```python
from build123d import *

# Parameters (mm, degrees)
SKETCH2_OUTSIDE_W = 12.738
SKETCH2_OUTSIDE_H = 12.738
EXTRUDE1_DEPTH    = 6
SKETCH3_R         = 2.125
EXTRUDE2_DEPTH    = 2
EXTRUDE2_TAPER    = 20
SKETCH4_R         = 1.35
EXTRUDE3_DEPTH    = 12
SKETCH5_W         = 1.5
SKETCH5_H         = 7.5
EXTRUDE4_DEPTH    = 0.75


with BuildPart() as part:
    # Sketch1 → Revolve1 (revolve)
    with BuildSketch(Plane.XY, mode=Mode.PRIVATE) as revolve1_sk:
        with BuildLine():
            Line((-6.597555333, -81.619969832), (-4.417555333, -81.619969832))
            ThreePointArc((-4.417555333, -81.619969832), (-4.276133977, -81.561391188), (-4.217555333, -81.419969832))
            Line((-4.217555333, -81.419969832), (-4.217555333, -80.780202359))
            ThreePointArc((-4.217555333, -80.780202359), (-4.241407579, -80.627613643), (-4.310688598, -80.489583262))
            Line((-4.310688598, -80.489583262), (-5.467555333, -78.869969832))
            Line((-5.467555333, -78.869969832), (-5.467555333, -72.569969832))
            Line((-5.467555333, -72.569969832), (-5.467555333, -68.619969832))
            Line((-5.467555333, -68.619969832), (-6.597555333, -68.619969832))
            Line((-6.597555333, -68.619969832), (-6.597555333, -81.619969832))
        make_face()
    revolve(revolve1_sk.sketch.rotate(Axis((-7.917555333, -68.619969832, 0), (0, -1, 0)), 180), axis=Axis((-7.917555333, -68.619969832, 0), (0, -1, 0)))

    # Sketch2 outside → Extrude1 (cut)
    with BuildSketch(Plane(origin=(0, -68.619969832, 0), x_dir=(-1, 0, 0), z_dir=(0, 1, 0))):
        with Locations((7.918, 0)):
            Rectangle(SKETCH2_OUTSIDE_W, SKETCH2_OUTSIDE_H)
        Polygon((5.301260243, 0), (7.917555333, -2.61629509), (10.533850424, 0), (7.917555333, 2.61629509), align=None, mode=Mode.SUBTRACT)
    extrude(amount=-EXTRUDE1_DEPTH, mode=Mode.SUBTRACT)

    # Sketch3 → Extrude2 (add)
    with BuildSketch(Plane(origin=(0, -74.619969832, 0), x_dir=(-1, 0, 0), z_dir=(0, 1, 0))):
        with Locations((7.917555333, 0)):
            Circle(SKETCH3_R)
    extrude(amount=EXTRUDE2_DEPTH, taper=EXTRUDE2_TAPER)

    # Sketch4 → Extrude3 (cut)
    with BuildSketch(Plane(origin=(0, -68.619969832, 0), x_dir=(-1, 0, 0), z_dir=(0, 1, 0))):
        with Locations((7.917555333, 0)):
            Circle(SKETCH4_R)
    extrude(amount=-EXTRUDE3_DEPTH, mode=Mode.SUBTRACT)

    # Sketch5 → Extrude4 (cut)
    with BuildSketch(Plane.XZ.offset(81.619969832)):
        with Locations((-7.917555333, 0)):
            Rectangle(SKETCH5_W, SKETCH5_H)
    extrude(amount=-EXTRUDE4_DEPTH, mode=Mode.SUBTRACT)


solid = part.part
```
Part model, mm, in its own coordinate system. A direction names the side the tool comes from. Round coordinates to 2 decimals unless told otherwise and drop trailing zeros. Write each loop counter-clockwise with the first axis right and the second up, starting at its lowest first coordinate (ties: lowest second). Pieces come first, ordered by that corner, then holes. Notation, with made-up numbers: (47.5, 86.25) -> (60.5, 86.25) arc R11 ccw to (60.5, 94.25) -> close; hole circle Ø8 at (-22.75, 48.25). An arc over 180 degrees is marked (long way). Return JSON: item names as keys, results as strings. Group by question number.
Q1. Pin check, flat tips, straight feed: pin 1 (0.8 mm diameter, centred on y = -81.5, z = -2.5, fed in from +X); pin 2 (1 mm diameter, centred on y = -80, z = 0.5, fed in from -X); pin 3 (1.5 mm diameter, centred on x = -7, y = -78, fed in from -Z). Stop position of each tip, or through.
Q2. Saw through at B-B on y = -77.5. Write the cut outline in (x, z).
Q3. Which spindle directions (+Z, -Z, +X, -X, +Y, -Y) get a long thin tool onto all of the face, cutting with end or side? Do faces 1 (the flat face through (-9.21, -71.578, -1.324)), 2 (the flat face through (-6.6, -71.6, -1.3)), 3 (the flat face through (-6.6, -71.6, 1.3)), 4 (the cylindrical face through (-5.47, -75.95, -0.11)), 5 (the flat face through (-8, -80.87, 2)). Say none if no direction does.
Q4. Saw through at C-C on y = -79.75. Write the cut outline in (x, z).
Q5. Mould opens along Z. For faces 6 (the conical face through (-6.482, -74.321, -1.415)), 7 (the cylindrical face through (-6.6, -81, -0.1)), 8 (the flat face through (-6.3, -74.62, -1.6)), 9 (the cylindrical face through (-9.205, -74.536, 0.406)) say: pulls with the +Z half, pulls with the -Z half, needs draft (parallel to the pull), parting line crosses it, or undercut.
Q6. Probe L1, parallel to Y at x = -8, z = 2.25; L2, parallel to X at y = -75.75, z = -0.75; L3, parallel to X at y = -71.75, z = -1. List the from-to ranges inside material, lowest first. Write a range as [from, to].
Answer:
{
 "1": {"pin 1": "x = -4.88", "pin 2": "x = -11.5", "pin 3": "z = -2.44"},
 "2": {"outline": "circle Ø4.9 at (-7.92, 0); hole circle Ø2.7 at (-7.92, 0)"},
 "3": {"face 1": "-Z, -X, +Y", "face 2": "-Z, +X, +Y", "face 3": "+Z, +X, +Y", "face 4": "+Y", "face 5": "+Z, -Z, -Y"},
 "4": {"outline": "circle Ø6.16 at (-7.92, 0); hole circle Ø2.7 at (-7.92, 0)"},
 "5": {"face 6": "pulls with the -Z half", "face 7": "undercut", "face 8": "needs draft", "face 9": "undercut"},
 "6": {"L1": "[-80.87, -68.62]", "L2": "[-10.25, -9.04], [-6.8, -5.59]", "L3": "[-9.53, -8.82], [-7.01, -6.3]"}
}
